Can you work these out from the model? Positions are in its coordinate system, mm. A direction names the side the tool comes from. Coordinates: 2 decimals unless noted, no trailing zeros. Order: outer loops, then holes, each group sorted by start corner. A loop starts at its lowest first (then second) coordinate and runs counter-clockwise, first axis right, second up. Notation, with made-up numbers: (75, 14.25) -> (90, 14.25) arc R31 ccw to (90, 39.25) -> close; hole circle Ø7 at (3.25, 69). An arc over 180 degrees is marked (long way). Use a Markdown table: item, result. Add a question column.
1. We'd pull the mould along X, two halves only. Please class faces 4 (the cylindrical face through (4.29, 6.83, 0.99)), 5 (the flat face through (0, 5.6, 4)), 6 (the flat face through (-3, -3.5, 1)): pulls with the +X half, pulls with the -X half, needs draft (parallel to the pull), parting line crosses it, or undercut.
2. Suppose I cut it at D-D, the plane x = 0. List the corners of the cut face in (y, z) for me, then the cut area to 3 significant figures.
3. Suppose I cut it at B-B, the plane y = -3.25. List the corners of the cut face in (x, z) for me, then the cut area to 3 significant figures.
4. Suppose I cut it at A-A, the plane z = 1.5. List the corners of the cut face in (x, y) for me, then the cut area to 3 significant figures.
5. For pin 1 Ø1 at (y, z) = (5.5, 5.5) entering from -X; pin 2 Ø0.6 at (x, z) = (3, 1) entering from -Y; pin 3 Ø1.3 at (x, z) = (0, 4) entering from -Y, each with a flat end and sliding along its axis, tell me the tip position at first contact or that it passes through.
6. If I drill on line 1 along Y through (x, z) = (-0.75, 3.25); line 2 along Y through (x, z) = (-1.5, 2.5); line 3 along X through (y, z) = (-3, 5.5), over which ranges is the centre line in solid material (lowest first)? Write a range as from..to.
7. Suppose I cut it at C-C, the plane z = 6.25. List the corners of the cut face in (x, y) for me, then the cut area to 3 significant figures.
8. For faces 1 (the flat face through (-3, 0, 1.3)), 2 (the flat face through (3.1, 0, 4)), 3 (the cylindrical face through (4.33, -6.79, 0.99)), which set-ups out of +Z, -Z, +X, -X, +Y, -Y let a thin tool reach every point of the face, with its end or its side?
```python
from build123d import *

# Parameters (mm, degrees)
CROQUIS1_W              = 9.2
CROQUIS1_H              = 4.2
SALIENTE_EXTRUIR1_DEPTH = 7
SALIENTE_EXTRUIR2_DEPTH = 2
SALIENTE_EXTRUIR3_START = 7
CROQUIS1_5_W            = 9.2
CROQUIS1_5_H            = 4.2
CROQUIS1_5_R            = 1.647263677
SALIENTE_EXTRUIR3_DEPTH = 1
SALIENTE_EXTRUIR4_START = 7
CROQUIS1_6_R            = 1.647263677
SALIENTE_EXTRUIR4_DEPTH = 7
CORTAR_EXTRUIR1_START   = -1.3
CROQUIS2_W              = 4.2
CROQUIS2_H              = 7
CROQUIS2_R              = 1.647263677
CROQUIS2_W_2            = 1.4
CORTAR_EXTRUIR1_DEPTH   = 1.3
REDONDEO1_R             = 0.5


with BuildPart() as part:
    # Croquis1 → Saliente-Extruir1 (new body)
    with BuildSketch(Plane(origin=(0, 0, 0), x_dir=(0, 1, 0), z_dir=(0, 0, 1))):
        with BuildLine():
            ThreePointArc((-5.6, 2.4), (-5.394974747, 2.894974747), (-4.9, 3.1))
            Line((-4.9, 3.1), (4.9, 3.1))
            ThreePointArc((4.9, 3.1), (5.394974747, 2.894974747), (5.6, 2.4))
            Line((5.6, 2.4), (5.6, -2.4))
            ThreePointArc((5.6, -2.4), (5.394974747, -2.894974747), (4.9, -3.1))
            Line((4.9, -3.1), (-4.9, -3.1))
            ThreePointArc((-4.9, -3.1), (-5.394974747, -2.894974747), (-5.6, -2.4))
            Line((-5.6, -2.4), (-5.6, 2.4))
        make_face()
        Rectangle(CROQUIS1_W, CROQUIS1_H, mode=Mode.SUBTRACT)
    extrude(amount=SALIENTE_EXTRUIR1_DEPTH)

    # Croquis1<4> → Saliente-Extruir2 (add)
    with BuildSketch(Plane(origin=(0, 0, 0), x_dir=(0, 1, 0), z_dir=(0, 0, 1))):
        with BuildLine():
            ThreePointArc((-4.9, -5.1), (-6.809188309, -4.309188309), (-7.6, -2.4))
            Line((-7.6, -2.4), (-7.6, 2.4))
            ThreePointArc((-7.6, 2.4), (-6.809188309, 4.309188309), (-4.9, 5.1))
            Line((-4.9, 5.1), (4.9, 5.1))
            ThreePointArc((4.9, 5.1), (6.809188309, 4.309188309), (7.6, 2.4))
            Line((7.6, 2.4), (7.6, -2.4))
            ThreePointArc((7.6, -2.4), (6.809188309, -4.309188309), (4.9, -5.1))
            Line((4.9, -5.1), (-4.9, -5.1))
        make_face()
        with BuildLine():
            Line((-5.6, -2.4), (-5.6, 2.4))
            ThreePointArc((-5.6, 2.4), (-5.394974747, 2.894974747), (-4.9, 3.1))
            Line((-4.9, 3.1), (4.9, 3.1))
            ThreePointArc((4.9, 3.1), (5.394974747, 2.894974747), (5.6, 2.4))
            Line((5.6, 2.4), (5.6, -2.4))
            ThreePointArc((5.6, -2.4), (5.394974747, -2.894974747), (4.9, -3.1))
            Line((4.9, -3.1), (-4.9, -3.1))
            ThreePointArc((-4.9, -3.1), (-5.394974747, -2.894974747), (-5.6, -2.4))
        make_face(mode=Mode.SUBTRACT)
    extrude(amount=SALIENTE_EXTRUIR2_DEPTH)

    # Croquis1<5> → Saliente-Extruir3 (add)
    with BuildSketch(Plane(origin=(0, 0, 0), x_dir=(0, 1, 0), z_dir=(0, 0, 1)).offset(SALIENTE_EXTRUIR3_START)):
        Rectangle(CROQUIS1_5_W, CROQUIS1_5_H)
        with Locations(Location((0, 0, 0), (0, 0, 270))):
            Circle(CROQUIS1_5_R, mode=Mode.SUBTRACT)
    extrude(amount=-SALIENTE_EXTRUIR3_DEPTH)

    # Croquis1<6> → Saliente-Extruir4 (add)
    with BuildSketch(Plane(origin=(0, 0, 0), x_dir=(0, 1, 0), z_dir=(0, 0, 1)).offset(SALIENTE_EXTRUIR4_START)):
        with Locations(Location((0, 0, 0), (0, 0, 270))):
            Circle(CROQUIS1_6_R)
    extrude(amount=-SALIENTE_EXTRUIR4_DEPTH)

    # Croquis2 → Cortar-Extruir1 (cut)
    # profile 1 of 3: a face of its own
    with BuildSketch(Plane(origin=(0, 0, 0), x_dir=(1, 0, 0), z_dir=(0, 0, -1)).offset(CORTAR_EXTRUIR1_START)):
        Rectangle(CROQUIS2_W, CROQUIS2_H)
        Circle(CROQUIS2_R, mode=Mode.SUBTRACT)
    # profile 2 of 3: a face of its own
    with BuildSketch(Plane(origin=(0, 0, 0), x_dir=(1, 0, 0), z_dir=(0, 0, -1)).offset(CORTAR_EXTRUIR1_START)):
        with Locations((-2.8, 0)):
            Rectangle(CROQUIS2_W_2, CROQUIS2_H)
    # profile 3 of 3: a face of its own
    with BuildSketch(Plane(origin=(0, 0, 0), x_dir=(1, 0, 0), z_dir=(0, 0, -1)).offset(CORTAR_EXTRUIR1_START)):
        with Locations((2.8, 0)):
            Rectangle(CROQUIS2_W_2, CROQUIS2_H)
    extrude(amount=CORTAR_EXTRUIR1_DEPTH, mode=Mode.SUBTRACT)

    # Redondeo1
    redondeo1_edges = [part.edges().sort_by_distance(p)[0] for p in [
        (0, -5.6, 7),
        (2.894974747, -5.394974747, 7),
        (3.1, 0, 7),
        (2.894974747, 5.394974747, 7),
        (0, 5.6, 7),
        (-2.894974747, 5.394974747, 7),
        (-3.1, 0, 7),
        (-2.894974747, -5.394974747, 7),
    ]]
    fillet(redondeo1_edges, radius=REDONDEO1_R)


solid = part.part
```
Worked out:
| question | item | result |
|---|---|---|
| 1 | face 4 | pulls with the +X half |
| 1 | face 5 | needs draft |
| 1 | face 6 | undercut |
| 2 | outline | (-7.6, 0) -> (-4.6, 0) -> (-4.6, 6) -> (-1.65, 6) -> (-1.65, 0) -> (1.65, 0) -> (1.65, 6) -> (4.6, 6) -> (4.6, 0) -> (7.6, 0) -> (7.6, 2) -> (5.6, 2) -> (5.6, 6.5) arc R0.5 ccw to (5.1, 7) -> (-5.1, 7) arc R0.5 ccw to (-5.6, 6.5) -> (-5.6, 2) -> (-7.6, 2) -> close |
| 2 | area | 50.9 mm² |
| 3 | outline | (-5.1, 0) -> (-3.5, 0) -> (-3.5, 1.3) -> (-2.1, 1.3) -> (-2.1, 6) -> (2.1, 6) -> (2.1, 1.3) -> (3.5, 1.3) -> (3.5, 0) -> (5.1, 0) -> (5.1, 2) -> (3.1, 2) -> (3.1, 6.5) arc R0.5 ccw to (2.6, 7) -> (-2.6, 7) arc R0.5 ccw to (-3.1, 6.5) -> (-3.1, 2) -> (-5.1, 2) -> close |
| 3 | area | 22.5 mm² |
| 4 | outline | (-5.1, -4.9) arc R2.7 ccw to (-2.4, -7.6) -> (2.4, -7.6) arc R2.7 ccw to (5.1, -4.9) -> (5.1, 4.9) arc R2.7 ccw to (2.4, 7.6) -> (-2.4, 7.6) arc R2.7 ccw to (-5.1, 4.9) -> close; circle Ø3.29 at (0, 0); hole (-2.1, -4.6) -> (2.1, -4.6) -> (2.1, 4.6) -> (-2.1, 4.6) -> close |
| 4 | area | 119 mm² |
| 5 | pin 1 | stops at x = -3.09 |
| 5 | pin 2 | stops at y = -7.58 |
| 5 | pin 3 | stops at y = -5.6 |
| 6 | line 1 | y = -5.6..-4.6, -1.47..1.47, 4.6..5.6 |
| 6 | line 2 | y = -5.6..-4.6, -0.68..0.68, 4.6..5.6 |
| 6 | line 3 | x = -3.1..-2.1, 2.1..3.1 |
| 7 | outline | (-3.1, -4.9) arc R0.7 ccw to (-2.4, -5.6) -> (2.4, -5.6) arc R0.7 ccw to (3.1, -4.9) -> (3.1, 4.9) arc R0.7 ccw to (2.4, 5.6) -> (-2.4, 5.6) arc R0.7 ccw to (-3.1, 4.9) -> close |
| 7 | area | 69.0 mm² |
| 8 | face 1 | -Z |
| 8 | face 2 | +Z, +X, +Y, -Y |
| 8 | face 3 | +Z, -Z, +X, -Y |
